from build123d import *

# Parameters (mm, degrees)
CABEZA_START            = -2.5
SK_CABEZA_R             = 2.25
CABEZA_DEPTH            = 2.5
SK_CUERPO_R             = 1.25
CUERPO_DEPTH            = 14
HEXAGONO_INTERIOR_START = -2.5
HEXAGONO_INTERIOR_DEPTH = 1.25


with BuildPart() as part:
    # Sk_Cabeza → Cabeza (new body)
    with BuildSketch(Plane.XY.offset(CABEZA_START)):
        Circle(SK_CABEZA_R)
    extrude(amount=CABEZA_DEPTH)

    # Sk_Cuerpo → Cuerpo (add)
    with BuildSketch(Plane.XY):
        Circle(SK_CUERPO_R)
    extrude(amount=CUERPO_DEPTH)

    # Sk_Hexagono_interior → Hexagono_interior (cut)
    with BuildSketch(Plane.XY.offset(HEXAGONO_INTERIOR_START)):
        Polygon((0, -1.154700538), (1, -0.577350269), (1, 0.577350269), (0, 1.154700538), (-1, 0.577350269), (-1, -0.577350269), align=None)
    extrude(amount=HEXAGONO_INTERIOR_DEPTH, mode=Mode.SUBTRACT)


solid = part.part
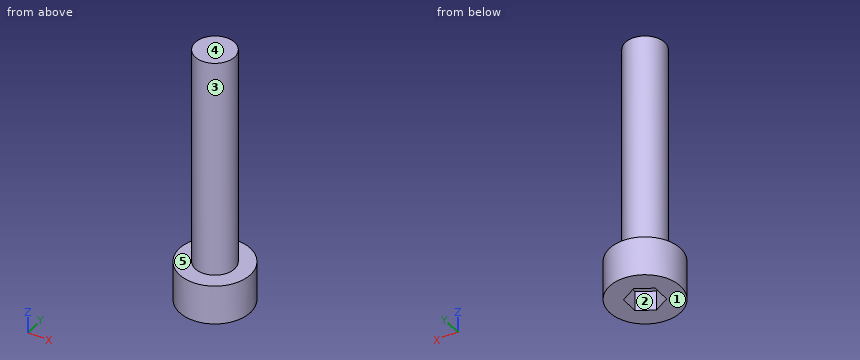
Work out the finished part from the listing and answer in its coordinate system (mm). Face numbers are marked on the shaded views. A direction names the side the tool comes from. Coordinates: 2 decimals unless noted, no trailing zeros. Order: outer loops, then holes, each group sorted by start corner. A loop starts at its lowest first (then second) coordinate and runs counter-clockwise, first axis right, second up. Notation, with made-up numbers: (81.5, -33) - (105.5, -33) arc R32 ccw to (105.5, -7) - close; hole circle Ø6 at (-16, -35). An arc over 180 degrees is marked (long way). Put each result on its own line as item: value. Start each with the question number.
1) Find the intervals of material crossed by line 1 (Z direction, x = -1.4, y = -1.1); line 2 (Y direction, x = -0.1, z = 3); line 3 (Z direction, x = 0.5, y = -0.4), in increasing order. Write a range as from..to.
2) Find section A-A (y = 0). Give the vertices of the cut face in (x, z).
3) For the marked faces 4 and 5, determine the directions among +Z, -Z, +X, -X, +Y, -Y from which every point of the face is accessible in a straight line to the end or side of a thin tool.
4) Flat-ended cylindrical pins translate along their axes: pin 1 (1 mm diameter, centred on x = -1.5, z = 4, fed in from -Y); pin 2 (0.6 mm diameter, centred on y = 0.5, z = -2, fed in from -X); pin 3 (1.5 mm diameter, centred on x = -0.5, y = 0, fed in from -Z); pin 4 (0.6 mm diameter, centred on y = 0.5, z = -2, fed in from +X). Find the tip coordinate at first contact, or state that the pin passes through.
5) Find section D-D (y = -1.75). Give the vertices of the cut face in (x, z).
6) For a pull along X with two mould halves and no side action, classify the marked faces 1, 2 and 3 as released by +X, released by -X, zero draft, split by the parting line, or undercut.
7) Find section B-B (z = 12). Give the vertices of the cut face in (x, y), plus the area to 3 significant figures.
8) Find section C-C (x = 0.85). Give the vertices of the cut face in (y, z).
Results list:
1. line 1: z = -2.5..0
1. line 2: y = -1.25..1.25
1. line 3: z = -1.25..14
2. outline: (-2.25, -2.5) - (-1, -2.5) - (-1, -1.25) - (1, -1.25) - (1, -2.5) - (2.25, -2.5) - (2.25, 0) - (1.25, 0) - (1.25, 14) - (-1.25, 14) - (-1.25, 0) - (-2.25, 0) - close
3. face 4: +Z, +X, -X, +Y, -Y
3. face 5: +Z
4. pin 1: stops at y = -0.75
4. pin 2: stops at x = -2.24
4. pin 3: stops at z = -2.5
4. pin 4: stops at x = 2.24
5. outline: (-1.41, -2.5) - (1.41, -2.5) - (1.41, 0) - (-1.41, 0) - close
6. face 1: zero draft
6. face 2: undercut
6. face 3: split by the parting line
7. outline: circle Ø2.5 at (0, 0)
7. area: 4.91 mm^2
8. outline: (-2.08, -2.5) - (-0.66, -2.5) - (-0.66, -1.25) - (0.66, -1.25) - (0.66, -2.5) - (2.08, -2.5) - (2.08, 0) - (0.92, 0) - (0.92, 14) - (-0.92, 14) - (-0.92, 0) - (-2.08, 0) - close
